from build123d import *

# Parameters (mm, degrees)
BOSS_EXTRUDE1_DEPTH = 6.604
FILLET1_R           = 12.7
CUT_EXTRUDE1_DEPTH  = 7.604
SKETCH3_W           = 6.35
SKETCH3_H           = 4.826
BOSS_EXTRUDE2_DEPTH = 6.604


with BuildPart() as part:
    # Sketch1 → Boss-Extrude1 (new body)
    with BuildSketch(Plane.XY):
        Polygon((-11.43, -1.905), (-11.43, -9.525), (6.985, -9.525), (6.985, 0), (12.7, 0), (12.7, -27.305), (-66.802, -27.305), (-66.802, -1.905), (-12.827, -1.905), align=None)
    extrude(amount=BOSS_EXTRUDE1_DEPTH)

    # Fillet1
    fillet1_edges = [part.edges().sort_by_distance(p)[0] for p in [
        (12.7, -27.305, 3.302),
        (-66.802, -27.305, 3.302),
    ]]
    fillet(fillet1_edges, radius=FILLET1_R)

    # Sketch2 → Cut-Extrude1 (cut, through all)
    with BuildSketch(Plane.XY.offset(6.604)):
        Polygon((-53.0098, -1.905), (-53.0098, -8.255), (-55.2958, -8.255), (-55.2958, -14.1986), (-53.0098, -14.1986), (-53.0098, -17.399), (-48.8442, -17.399), (-48.8442, -14.1986), (-46.5582, -14.1986), (-46.5582, -8.255), (-48.8442, -8.255), (-48.8442, -1.905), align=None)
        Polygon((-33.9598, -1.905), (-33.9598, -8.255), (-36.2458, -8.255), (-36.2458, -14.1986), (-33.9598, -14.1986), (-33.9598, -17.399), (-29.7942, -17.399), (-29.7942, -14.1986), (-27.5082, -14.1986), (-27.5082, -8.255), (-29.7942, -8.255), (-29.7942, -1.905), align=None)
    extrude(amount=-CUT_EXTRUDE1_DEPTH, mode=Mode.SUBTRACT)

    # Sketch3 → Boss-Extrude2 (add)
    with BuildSketch(Plane.XY.offset(6.604)):
        with Locations((-60.452, 0.508)):
            Rectangle(SKETCH3_W, SKETCH3_H)
        with Locations((-41.402, 0.508)):
            Rectangle(SKETCH3_W, SKETCH3_H)
        with Locations((-22.352, 0.508)):
            Rectangle(SKETCH3_W, SKETCH3_H)
    extrude(amount=-BOSS_EXTRUDE2_DEPTH)


solid = part.part
The listing builds one solid part. Answer for the finished solid, in the listing's coordinates (mm). A direction names the side the tool comes from. Coordinates: 2 decimals unless noted, no trailing zeros. Write each loop counter-clockwise with the first axis right and the second up, starting at its lowest first coordinate (ties: lowest second). Pieces come first, ordered by that corner, then holes. Notation, with made-up numbers: M -21,-22.5 L 13,-22.5 A12 cw 13,-13.5 Z; hole C 23,50.25 d1. An arc over 180 degrees is marked long. Write each question's results on one line, items separated by ' | '.
Item 1: The part is cut by section A-A on y = -10.5. Determine the outline of the cut face in (x, z).
Answer below:
outline: M -66.8,0 L -55.3,0 L -55.3,6.6 L -66.8,6.6 Z; M -46.56,0 L -36.25,0 L -36.25,6.6 L -46.56,6.6 Z; M -27.51,0 L 12.7,0 L 12.7,6.6 L -27.51,6.6 Z
Item 2: For a pull along Y with two mould halves and no side action, classify faces 1 (the face through (10, 0, 3)), 2 (the face through (6.985, -5, 3)), 3 (the face through (-36.246, -11, 3)) as released by +Y, released by -Y, zero draft, split by the parting line, or undercut.
Answer below:
face 1: released by +Y | face 2: zero draft | face 3: undercut
Item 3: Given P1, Ø0.7, axis at x = -54.5, z = 3.5, coming from the +Y side (3 decimals); P2, Ø2.5, axis at y = 0, z = 3.5, coming from the -X side; P3, Ø2, axis at x = -31.5, z = 2.5, coming from the +Y side, each flat-ended and moving along its own axis, determine where each tip first touches the part or whether it passes through.
Answer below:
P1: y = -1.905 | P2: x = -63.63 | P3: y = -17.4
Item 4: The part is cut by section D-D on y = 1. Determine the outline of the cut face in (x, z), and give its area (3 significant figures).
Answer below:
outline: M -63.63,0 L -57.28,0 L -57.28,6.6 L -63.63,6.6 Z; M -44.58,0 L -38.23,0 L -38.23,6.6 L -44.58,6.6 Z; M -25.53,0 L -19.18,0 L -19.18,6.6 L -25.53,6.6 Z | area: 126 mm2
Item 5: The part is cut by section C-C on x = -52. Determine the outline of the cut face in (y, z) (3 decimals).
Answer below:
outline: M -27.305,0 L -17.399,0 L -17.399,6.604 L -27.305,6.604 Z
Item 6: The part is cut by section B-B on y = -7. Determine the outline of the cut face in (x, z) (3 decimals).
Answer below:
outline: M -66.802,0 L -53.01,0 L -53.01,6.604 L -66.802,6.604 Z; M -48.844,0 L -33.96,0 L -33.96,6.604 L -48.844,6.604 Z; M -29.794,0 L -11.43,0 L -11.43,6.604 L -29.794,6.604 Z; M 6.985,0 L 12.7,0 L 12.7,6.604 L 6.985,6.604 Z
Item 7: Consider probe 1 along X at (y, z) = (-5.5, 2.25) (3 decimals); probe 2 along X at (y, z) = (-10, 5); probe 3 along X at (y, z) = (0.5, 5.5). Determine where each line is inside the solid, lowest interval first. Write a range as [from, to].
Answer below:
probe 1: [-66.802, -53.01], [-48.844, -33.96], [-29.794, -11.43], [6.985, 12.7] | probe 2: [-66.8, -55.3], [-46.56, -36.25], [-27.51, 12.7] | probe 3: [-63.63, -57.28], [-44.58, -38.23], [-25.53, -19.18]
Item 8: Which of the six approach directions +Z, -Z, +X, -X, +Y, -Y give full straight-line access (tool end or side, diameter ignored) to faces 4 (the face through (-29, -14.199, 3)), 5 (the face through (12.7, -7, 3)), 6 (the face through (-25.527, 0, 3)), 7 (the face through (-65, -1.905, 3))?
Answer below:
face 4: +Z, -Z | face 5: +Z, -Z, +X, +Y, -Y | face 6: +Z, -Z, +Y | face 7: +Z, -Z, -X, +Y
